from build123d import *

# Parameters (mm, degrees)
SKETCH_1_R      = 5.0225
SKETCH_1_R_2    = 2
EXTRUDE_1_DEPTH = 4
FILLET_1_R      = 2
FILLET_2_R      = 1.3


with BuildPart() as part:
    # 草图1 → 凸台-拉伸1 (new body)
    with BuildSketch(Plane.XY):
        with BuildLine():
            Line((298.551498293, -96.645689396), (302.551498293, -96.645689396))
            Line((302.551498293, -96.645689396), (302.551498293, -98.644151028))
            Line((302.551498293, -98.644151028), (305.251498293, -98.644151028))
            Line((305.251498293, -98.644151028), (305.251498293, -96.645689396))
            Line((305.251498293, -96.645689396), (307.951498293, -96.645689396))
            Line((307.951498293, -96.645689396), (307.951498293, -93.645689396))
            Line((307.951498293, -93.645689396), (305.251498293, -93.645689396))
            Line((305.251498293, -93.645689396), (305.251498293, -91.647227763))
            Line((305.251498293, -91.647227763), (302.551498293, -91.647227763))
            Line((302.551498293, -91.647227763), (302.551498293, -93.645689396))
            Line((302.551498293, -93.645689396), (298.551498293, -93.645689396))
            Line((298.551498293, -93.645689396), (298.551498293, -84.145716775))
            Line((298.551498293, -84.145716775), (293.551498293, -84.145716775))
            Line((293.551498293, -84.145716775), (293.551498293, -76.145716775))
            Line((293.551498293, -76.145716775), (298.551498293, -76.145716775))
            Line((298.551498293, -76.145716775), (298.551498293, -66.645694374))
            Line((298.551498293, -66.645694374), (302.551498293, -66.645694374))
            Line((302.551498293, -66.645694374), (302.551498293, -68.644156006))
            Line((302.551498293, -68.644156006), (305.251498293, -68.644156006))
            Line((305.251498293, -68.644156006), (305.251498293, -66.645694374))
            Line((305.251498293, -66.645694374), (307.951498293, -66.645694374))
            Line((307.951498293, -66.645694374), (307.951498293, -63.645694374))
            Line((307.951498293, -63.645694374), (305.251498293, -63.645694374))
            Line((305.251498293, -63.645694374), (305.251498293, -61.647232741))
            Line((305.251498293, -61.647232741), (302.551498293, -61.647232741))
            Line((302.551498293, -61.647232741), (302.551498293, -63.645694374))
            Line((302.551498293, -63.645694374), (298.551498293, -63.645694374))
            Line((298.551498293, -63.645694374), (298.551498293, -54.145671973))
            Line((298.551498293, -54.145671973), (293.551498293, -54.145671973))
            Line((293.551498293, -54.145671973), (293.551498293, -46.145671973))
            Line((293.551498293, -46.145671973), (298.551498293, -46.145671973))
            Line((298.551498293, -46.145671973), (298.551498293, -35.045714286))
            Line((298.551498293, -35.045714286), (307.942857143, -35.045714286))
            Line((307.942857143, -35.045714286), (321.159325739, 4.854285714))
            ThreePointArc((321.159325739, 4.854285714), (348.542857143, 32.081451417), (375.926388547, 4.854285714))
            Line((375.926388547, 4.854285714), (376.364473934, -71.645714286))
            Line((376.364473934, -71.645714286), (324.194731876, -140.145734198))
            Line((324.194731876, -140.145734198), (298.551498293, -140.145734198))
            Line((298.551498293, -140.145734198), (298.551498293, -126.645734198))
            Line((298.551498293, -126.645734198), (302.551498293, -126.645734198))
            Line((302.551498293, -126.645734198), (302.551498293, -128.644195831))
            Line((302.551498293, -128.644195831), (305.251498293, -128.644195831))
            Line((305.251498293, -128.644195831), (305.251498293, -126.645734198))
            Line((305.251498293, -126.645734198), (307.951498293, -126.645734198))
            Line((307.951498293, -126.645734198), (307.951498293, -123.645734198))
            Line((307.951498293, -123.645734198), (305.251498293, -123.645734198))
            Line((305.251498293, -123.645734198), (305.251498293, -121.647272565))
            Line((305.251498293, -121.647272565), (302.551498293, -121.647272565))
            Line((302.551498293, -121.647272565), (302.551498293, -123.645734198))
            Line((302.551498293, -123.645734198), (298.551498293, -123.645734198))
            Line((298.551498293, -123.645734198), (298.551498293, -114.145711797))
            Line((298.551498293, -114.145711797), (293.551498293, -114.145711797))
            Line((293.551498293, -114.145711797), (293.551498293, -106.145711797))
            Line((293.551498293, -106.145711797), (298.551498293, -106.145711797))
            Line((298.551498293, -106.145711797), (298.551498293, -96.645689396))
        make_face()
        with Locations((348.542857143, 4.854285714)):
            Circle(SKETCH_1_R, mode=Mode.SUBTRACT)
        with Locations((348.542857143, 24.697471009)):
            Circle(SKETCH_1_R_2, mode=Mode.SUBTRACT)
        with Locations((320.551498293, -134.145734198)):
            Circle(SKETCH_1_R_2, mode=Mode.SUBTRACT)
        with Locations((370.364473934, -65.645714286)):
            Circle(SKETCH_1_R_2, mode=Mode.SUBTRACT)
        with Locations((313.942857143, -41.045714286)):
            Circle(SKETCH_1_R_2, mode=Mode.SUBTRACT)
        Polygon((354.95315454, -69.835495731), (328.585486884, -106.094838527), (325.087312939, -56.813896117), align=None, mode=Mode.SUBTRACT)
        Polygon((329.57699596, -36.9530828), (354.34318526, -47.751218186), (344.764617274, -16.87417598), align=None, mode=Mode.SUBTRACT)
    extrude(amount=EXTRUDE_1_DEPTH)

    # 圆角1
    fillet_1_edges = [part.edges().sort_by_distance(p)[0] for p in [
        (354.95315454, -69.835495731, 2),
        (325.087312939, -56.813896117, 2),
        (328.585486884, -106.094838527, 2),
        (344.764617274, -16.87417598, 2),
        (329.57699596, -36.9530828, 2),
        (354.34318526, -47.751218186, 2),
    ]]
    fillet(fillet_1_edges, radius=FILLET_1_R)

    # 圆角2
    fillet_2_edges = [part.edges().sort_by_distance(p)[0] for p in [
        (293.551498293, -114.145711797, 2),
        (293.551498293, -106.145711797, 2),
        (293.551498293, -84.145716775, 2),
        (293.551498293, -76.145716775, 2),
        (293.551498293, -54.145671973, 2),
        (293.551498293, -46.145671973, 2),
    ]]
    fillet(fillet_2_edges, radius=FILLET_2_R)


solid = part.part
Geometry check sheet. Reference: the model listing, model coordinates, mm. A direction names the side the tool comes from. Give positions to 0.01 mm unless a question says otherwise; leave off trailing zeros. Order: outer loops, then holes, each group sorted by start corner. A loop starts at its lowest first (then second) coordinate and runs counter-clockwise, first axis right, second up.
1) Draft check along Y on faces 5 (the cylindrical face through (347.943, 32.075, 1.972)), 6 (the cylindrical face through (353.333, 6.363, 1.972)), 7 (the flat face through (336, -53, 4)). Enter one of: released by +Y, released by -Y, zero draft, split by the parting line, or undercut.
Results are:
face 5: released by +Y
face 6: undercut
face 7: zero draft
2) Cross-section at C-C (z = 0.9). Give the number of separate pieces and of enclosed holes in the cut face, then the cut area to 3 significant figures.
Results are:
separate pieces: 1
enclosed holes: 7
area: 8,860 mm2
3) Material ranges on probe 1 along Y at (x, z) = (299, 3.05); probe 2 along Y at (x, z) = (304, 1.15); probe 3 along X at (y, z) = (-66.5, 2.1) (1 decimal), recorded low to high.
Results are:
probe 1: y = -140.15 to -126.65, -123.65 to -96.65, -93.65 to -66.65, -63.65 to -35.05
probe 2: y = -140.15 to -128.64, -121.65 to -98.64, -91.65 to -68.64, -61.65 to -35.05
probe 3: x = 308 to 325.8, 347.3 to 368.6, 372.2 to 376.3
4) Tool access check on faces 1 (the flat face through (349.534, -32.249, 1.972)), 2 (the flat face through (298.551, -133, 2)), 3 (the flat face through (297, -46.146, 2)), 4 (the flat face through (297, -76.146, 2)). Record the directions out of +Z, -Z, +X, -X, +Y, -Y that give a thin tool (end or side, any length) a straight path to the whole face; none if there is none.
Results are:
face 1: +Z, -Z
face 2: +Z, -Z, -X, -Y
face 3: +Z, -Z, -X, +Y
face 4: +Z, -Z, -X
5) Gauge pin test, flat ends, axial feed: pin 1 (1 mm diameter, centred on x = 347.5, z = 3, fed in from -Y); pin 2 (1 mm diameter, centred on y = -98, z = 1, fed in from +X); pin 3 (1.8 mm diameter, centred on x = 296.5, z = 1.5, fed in from -Y). Record the tip position at first contact, or that the pin passes through.
Results are:
pin 1: stops at y = -110.2
pin 2: stops at x = 356.67
pin 3: stops at y = -114.15
6) Cross-section at A-A (y = 7.5). Record the boundary of the cut face in (x, z).
Results are:
outline: (321.3, 0) - (344.27, 0) - (344.27, 4) - (321.3, 4) - close; (352.81, 0) - (375.78, 0) - (375.78, 4) - (352.81, 4) - close
7) Cross-section at B-B (y = -27). Record the boundary of the cut face in (x, z).
Results are:
outline: (310.61, 0) - (337.11, 0) - (337.11, 4) - (310.61, 4) - close; (347.91, 0) - (376.11, 0) - (376.11, 4) - (347.91, 4) - close
